from build123d import *

# Parameters (mm, degrees)
F0_W           = 12.7
F0_H           = 76.2
F1_DEPTH       = 76.2
F3_D           = 6.35
F3_CBORE_D     = 9.525
F3_CBORE_DEPTH = 6.35
F4_R           = 10


with BuildPart() as f1:
    # F0 (on Front) → F1 (new body)
    with BuildSketch(Plane.XZ):
        Rectangle(F0_W, F0_H)
    extrude(amount=F1_DEPTH)

    # F3 (through all)
    with Locations(Plane.XY.offset(38.1)):
        with Locations((0, -38.1)):
            CounterBoreHole(F3_D / 2, F3_CBORE_D / 2, F3_CBORE_DEPTH)

    # F4
    f4_edges = [f1.edges().sort_by_distance(p)[0] for p in [
        (0, -76.2, 38.1),
        (0, 0, 38.1),
    ]]
    fillet(f4_edges, radius=F4_R)


solid = f1.part
Input: part model. Units: mm. Frame: model coordinates. Coordinates: 2 decimals unless noted, no trailing zeros. Loops run counter-clockwise (first coordinate to the right, second up) from the corner with the lowest first, then second, coordinate; pieces in that order, holes last.
(1) Section C-C on z = 19.5. Return the cut outline in (x, y) (3 decimals).
(2) Pull-direction query (Y, two-part tool) for faces 1 (the face through (4, -38, -38.1)), 2 (the face through (2.198, -42.325, 34.969)), 3 (the face through (0, 0, -5)); classes: released by +Y, released by -Y, zero draft, split by the parting line, or undercut.
(3) First-contact query: pin 1 Ø3 at (x, y) = (-1, -39.5) entering from +Z. Flat tip, straight axial feed; report the tip coordinate or a pass-through.
(4) Material intervals for probe 1 along X at (y, z) = (-38, 24.5); probe 2 along X at (y, z) = (-38, 34); probe 3 along Y at (x, z) = (-2.75, 29), sorted ascending.
Data:
1. outline: (-6.35, -76.2) - (6.35, -76.2) - (6.35, 0) - (-6.35, 0) - close; hole circle Ø6.35 at (0, -38.1)
2. face 1: zero draft
2. face 2: undercut
2. face 3: released by +Y
3. pin 1: stops at z = 31.75
4. probe 1: x = -6.35 to -3.17, 3.17 to 6.35
4. probe 2: x = -6.35 to -4.76, 4.76 to 6.35
4. probe 3: y = -76.16 to -39.69, -36.51 to -0.04
